Build history of the part. All positions in model axes, mm. A direction names the side the tool comes from. Coordinates: 2 decimals unless noted, no trailing zeros. Loops run counter-clockwise (first coordinate to the right, second up) from the corner with the lowest first, then second, coordinate; pieces in that order, holes last.
(1) Slice it at A-A (y = 8.25). Give the cut face in (x, z), and give its area (3 significant figures).
(2) Two-plate mould, pull along Z, no slides. Class faces 1 (the face through (35, 6, -72)), 2 (the face through (35, 1, -52)), 3 (the face through (3, 12, -37)): pulls with the +Z half, pulls with the -Z half, needs draft (parallel to the pull), parting line crosses it, or undercut.
(3) Flat gauge pin, fed straight in: P1, Ø8, axis at x = 47.5, z = -16.5, coming from the +Y side. Where does the tip first touch, or does it go through?
(4) Slice it at B-B (x = 51). Give the cut face in (y, z).
(5) Slice it at D-D (z = -59.5). Give the cut face in (x, y).
(6) Wall check: L1, parallel to Z at x = 51.5, y = 6.75; L2, parallel to Z at x = 11, y = 1.5; L3, parallel to X at y = 4.25, z = -49. Give the ranges that are in metal, low to high.
(7) Tool access for faces 4 (the face through (60, 6, -36)), 5 (the face through (35, 1, -20)), 6 (the face through (35, 6, 0)): list every direction of +Z, -Z, +X, -X, +Y, -Y with a clear straight run to the whole face (end or side of a thin tool).
(8) Slice it at C-C (z = -27.5). Give the cut face in (x, y), and give its area (3 significant figures).
from build123d import *

# Parameters (mm, degrees)
SKETCH1_W           = 70
SKETCH1_H           = 72
BOSS_EXTRUDE1_DEPTH = 2
SKETCH2_W           = 50
SKETCH2_H           = 32
CUT_EXTRUDE1_DEPTH  = 12
SKETCH3_W           = 10
SKETCH3_H           = 52
SKETCH3_H_2         = 10
SKETCH3_W_2         = 50
BOSS_EXTRUDE2_DEPTH = 10


with BuildPart() as part:
    # Sketch1 → Boss-Extrude1 (new body)
    with BuildSketch(Plane(origin=(0, 0, 0), x_dir=(1, 0, 0), z_dir=(0, 1, 0))):
        with Locations((35, 36)):
            Rectangle(SKETCH1_W, SKETCH1_H)
    extrude(amount=BOSS_EXTRUDE1_DEPTH)

    # Sketch2 → Cut-Extrude1 (cut)
    with BuildSketch(Plane(origin=(0, 2, 0), x_dir=(1, 0, 0), z_dir=(0, 1, 0))):
        with Locations((35, 36)):
            Rectangle(SKETCH2_W, SKETCH2_H)
    extrude(amount=-CUT_EXTRUDE1_DEPTH, mode=Mode.SUBTRACT)

    # Sketch3 → Boss-Extrude2 (add)
    with BuildSketch(Plane(origin=(0, 2, 0), x_dir=(1, 0, 0), z_dir=(0, 1, 0))):
        with Locations((5, 36)):
            Rectangle(SKETCH3_W, SKETCH3_H)
        with Locations((5, 67)):
            Rectangle(SKETCH3_W, SKETCH3_H_2)
        with Locations((35, 67)):
            Rectangle(SKETCH3_W_2, SKETCH3_H_2)
        with Locations((5, 5)):
            Rectangle(SKETCH3_W, SKETCH3_H_2)
        with Locations((35, 5)):
            Rectangle(SKETCH3_W_2, SKETCH3_H_2)
        with Locations((65, 5)):
            Rectangle(SKETCH3_W, SKETCH3_H_2)
        with Locations((65, 36)):
            Rectangle(SKETCH3_W, SKETCH3_H)
        with Locations((65, 67)):
            Rectangle(SKETCH3_W, SKETCH3_H_2)
    extrude(amount=BOSS_EXTRUDE2_DEPTH)


solid = part.part
Response values:
1. outline: (0, -72) - (70, -72) - (70, 0) - (0, 0) - close; hole (10, -62) - (60, -62) - (60, -10) - (10, -10) - close
1. area: 2,440 mm2
2. face 1: pulls with the -Z half
2. face 2: undercut
2. face 3: needs draft
3. P1: stops at y = 2
4. outline: (0, -72) - (12, -72) - (12, -62) - (2, -62) - (2, -52) - (0, -52) - close; (0, -20) - (2, -20) - (2, -10) - (12, -10) - (12, 0) - (0, 0) - close
5. outline: (0, 0) - (70, 0) - (70, 12) - (60, 12) - (60, 2) - (10, 2) - (10, 12) - (0, 12) - close
6. L1: z = -72 to -62, -10 to 0
6. L2: z = -72 to -52, -20 to 0
6. L3: x = 0 to 10, 60 to 70
7. face 4: +Y
7. face 5: +Y, -Y
7. face 6: +Z, +X, -X, +Y, -Y
8. outline: (0, 0) - (10, 0) - (10, 12) - (0, 12) - close; (60, 0) - (70, 0) - (70, 12) - (60, 12) - close
8. area: 240 mm2
